from build123d import *

# Parameters (mm, degrees)
SKETCH2_R           = 145
SKETCH2_R_2         = 105
BOSS_EXTRUDE1_START = -50
SKETCH3_W           = 360
SKETCH3_H           = 360
SKETCH3_R           = 145
BOSS_EXTRUDE1_DEPTH = 50
FILLET1_R           = 20
SKETCH4_W           = 360
SKETCH4_H           = 360
SKETCH4_R           = 145
BOSS_EXTRUDE2_DEPTH = 50
FILLET2_R           = 20
SKETCH5_R           = 30
CUT_EXTRUDE1_DEPTH  = 10
CUT_EXTRUDE2_REACH  = 734.735
SKETCH6_R           = 15
CUT_EXTRUDE3_DEPTH  = 10
CUT_EXTRUDE4_REACH  = 848.699
SKETCH8_R           = 15
CIRPATTERN1_COUNT   = 4
CHAMFER1_SIZE       = 10
CHAMFER2_SIZE       = 10


with BuildPart() as part:
    # Sweep-Thin1: sweep along a path in Sketch1
    with BuildLine(Plane.XY) as sweep_thin1_path:
        Line((0, 0), (-150, 0))
        ThreePointArc((-150, 0), (-333.847763109, 76.152236891), (-410, 260))
        Line((-410, 260), (-410, 410))
    # Sketch2 → Sweep-Thin1 (sweep)
    with BuildSketch(Plane(origin=(0, 0, 0), x_dir=(0, 0, -1), z_dir=(1, 0, 0))):
        Circle(SKETCH2_R)
        Circle(SKETCH2_R_2, mode=Mode.SUBTRACT)
    sweep(path=sweep_thin1_path.line)

    # Sketch3 → Boss-Extrude1 (add)
    with BuildSketch(Plane(origin=(0, 0, 0), x_dir=(0, 0, -1), z_dir=(1, 0, 0)).offset(BOSS_EXTRUDE1_START)):
        Rectangle(SKETCH3_W, SKETCH3_H)
        with Locations(Location((0, 0, 0), (0, 0, 270))):
            Circle(SKETCH3_R, mode=Mode.SUBTRACT)
    extrude(amount=BOSS_EXTRUDE1_DEPTH)

    # Fillet1
    fillet1_edges = [part.edges().sort_by_distance(p)[0] for p in [
        (-25, -180, -180),
        (-25, -180, 180),
        (-25, 180, 180),
        (-25, 180, -180),
    ]]
    fillet(fillet1_edges, radius=FILLET1_R)

    # Sketch4 → Boss-Extrude2 (add)
    with BuildSketch(Plane(origin=(0, 410, 0), x_dir=(1, 0, 0), z_dir=(0, 1, 0))):
        with Locations((-410, 0)):
            Rectangle(SKETCH4_W, SKETCH4_H)
        with Locations(Location((-410, 0, 0), (0, 0, 180))):
            Circle(SKETCH4_R, mode=Mode.SUBTRACT)
    extrude(amount=-BOSS_EXTRUDE2_DEPTH)

    # Fillet2
    fillet2_edges = [part.edges().sort_by_distance(p)[0] for p in [
        (-230, 385, -180),
        (-230, 385, 180),
        (-590, 385, 180),
        (-590, 385, -180),
    ]]
    fillet(fillet2_edges, radius=FILLET2_R)

    # Sketch5 → Cut-Extrude1 (cut)
    with BuildSketch(Plane(origin=(0, 0, 0), x_dir=(0, 0, -1), z_dir=(1, 0, 0))):
        with Locations((-130, 130)):
            Circle(SKETCH5_R)
        with Locations((130, 130)):
            Circle(SKETCH5_R)
        with Locations((-130, -130)):
            Circle(SKETCH5_R)
        with Locations((130, -130)):
            Circle(SKETCH5_R)
    extrude(amount=-CUT_EXTRUDE1_DEPTH, mode=Mode.SUBTRACT)

    # Sketch6 → Cut-Extrude2 (cut, up to next)
    with BuildSketch(Plane(origin=(-10, 0, 0), x_dir=(0, 0, -1), z_dir=(1, 0, 0)), mode=Mode.PRIVATE) as cut_extrude2_sk1:
        with Locations((-130, 130)):
            Circle(SKETCH6_R)
    cut_extrude2_tool1 = extrude(cut_extrude2_sk1.sketch, amount=-CUT_EXTRUDE2_REACH, mode=Mode.PRIVATE) & part.part
    # Sketch6 → Cut-Extrude2 (cut, up to next)
    with BuildSketch(Plane(origin=(-10, 0, 0), x_dir=(0, 0, -1), z_dir=(1, 0, 0)), mode=Mode.PRIVATE) as cut_extrude2_sk2:
        with Locations(Location((130, 130, 0), (0, 0, 180))):
            Circle(SKETCH6_R)
    cut_extrude2_tool2 = extrude(cut_extrude2_sk2.sketch, amount=-CUT_EXTRUDE2_REACH, mode=Mode.PRIVATE) & part.part
    # Sketch6 → Cut-Extrude2 (cut, up to next)
    with BuildSketch(Plane(origin=(-10, 0, 0), x_dir=(0, 0, -1), z_dir=(1, 0, 0)), mode=Mode.PRIVATE) as cut_extrude2_sk3:
        with Locations((130, -130)):
            Circle(SKETCH6_R)
    cut_extrude2_tool3 = extrude(cut_extrude2_sk3.sketch, amount=-CUT_EXTRUDE2_REACH, mode=Mode.PRIVATE) & part.part
    # Sketch6 → Cut-Extrude2 (cut, up to next)
    with BuildSketch(Plane(origin=(-10, 0, 0), x_dir=(0, 0, -1), z_dir=(1, 0, 0)), mode=Mode.PRIVATE) as cut_extrude2_sk4:
        with Locations(Location((-130, -130, 0), (0, 0, 180))):
            Circle(SKETCH6_R)
    cut_extrude2_tool4 = extrude(cut_extrude2_sk4.sketch, amount=-CUT_EXTRUDE2_REACH, mode=Mode.PRIVATE) & part.part
    add(cut_extrude2_tool1.solids().sort_by_distance((-10, 130, 130))[0], mode=Mode.SUBTRACT)
    add(cut_extrude2_tool2.solids().sort_by_distance((-10, 130, -130))[0], mode=Mode.SUBTRACT)
    add(cut_extrude2_tool3.solids().sort_by_distance((-10, -130, -130))[0], mode=Mode.SUBTRACT)
    add(cut_extrude2_tool4.solids().sort_by_distance((-10, -130, 130))[0], mode=Mode.SUBTRACT)

    # Sketch7 → Cut-Extrude3 (cut)
    with BuildSketch(Plane(origin=(0, 410, 0), x_dir=(1, 0, 0), z_dir=(0, 1, 0))):
        with BuildLine():
            Line((-540, 100), (-540, 130))
            Line((-540, 130), (-510, 130))
            ThreePointArc((-510, 130), (-561.213203436, 151.213203436), (-540, 100))
        make_face()
        with BuildLine():
            Line((-510, 130), (-540, 130))
            Line((-540, 130), (-540, 100))
            ThreePointArc((-540, 100), (-518.786796564, 108.786796564), (-510, 130))
        make_face()
        with BuildLine():
            ThreePointArc((-250, 130), (-280, 160), (-310, 130))
            Line((-310, 130), (-280, 130))
            Line((-280, 130), (-280, 100))
            ThreePointArc((-280, 100), (-258.786796564, 108.786796564), (-250, 130))
        make_face()
        with BuildLine():
            Line((-280, 130), (-310, 130))
            ThreePointArc((-310, 130), (-301.213203436, 108.786796564), (-280, 100))
            Line((-280, 100), (-280, 130))
        make_face()
        with BuildLine():
            ThreePointArc((-250, -130), (-258.786796564, -108.786796564), (-280, -100))
            Line((-280, -100), (-280, -130))
            Line((-280, -130), (-310, -130))
            ThreePointArc((-310, -130), (-280, -160), (-250, -130))
        make_face()
        with BuildLine():
            Line((-280, -130), (-280, -100))
            ThreePointArc((-280, -100), (-301.213203436, -108.786796564), (-310, -130))
            Line((-310, -130), (-280, -130))
        make_face()
        with BuildLine():
            ThreePointArc((-510, -130), (-518.786796564, -108.786796564), (-540, -100))
            Line((-540, -100), (-540, -130))
            Line((-540, -130), (-510, -130))
        make_face()
        with BuildLine():
            Line((-540, -130), (-540, -100))
            ThreePointArc((-540, -100), (-561.213203436, -151.213203436), (-510, -130))
            Line((-510, -130), (-540, -130))
        make_face()
    extrude(amount=-CUT_EXTRUDE3_DEPTH, mode=Mode.SUBTRACT)

    # Sketch8 → Cut-Extrude4 (cut, up to next)
    with BuildSketch(Plane(origin=(0, 400, 0), x_dir=(1, 0, 0), z_dir=(0, 1, 0)), mode=Mode.PRIVATE) as cut_extrude4_sk1:
        with Locations(Location((-540, 130, 0), (0, 0, 180))):
            Circle(SKETCH8_R)
    cut_extrude4_tool1 = extrude(cut_extrude4_sk1.sketch, amount=-CUT_EXTRUDE4_REACH, mode=Mode.PRIVATE) & part.part
    cut_extrude4 = cut_extrude4_tool1.solids().sort_by_distance((-540, 400, -130))[0]
    add(cut_extrude4, mode=Mode.SUBTRACT)

    # CirPattern1: Cut-Extrude4 ×4 about axis
    cirpattern1_axis = Axis((-410, 0, 0), (0, 1, 0))
    for i in range(1, CIRPATTERN1_COUNT):
        add(cut_extrude4.rotate(cirpattern1_axis, i * 360 / CIRPATTERN1_COUNT), mode=Mode.SUBTRACT)

    # Chamfer1
    chamfer1_edges = [part.edges().sort_by_distance(p)[0] for p in [
        (0, 0, 105),
    ]]
    chamfer(chamfer1_edges, length=CHAMFER1_SIZE)

    # Chamfer2
    chamfer2_edges = [part.edges().sort_by_distance(p)[0] for p in [
        (-410, 410, 105),
    ]]
    chamfer(chamfer2_edges, length=CHAMFER2_SIZE)


solid = part.part
Can you work these out from the model? Positions are in its coordinate system, mm. A direction names the side the tool comes from. Give positions to 0.01 mm unless a question says otherwise; leave off trailing zeros. Write each loop counter-clockwise with the first axis right and the second up, starting at its lowest first coordinate (ties: lowest second). Pieces come first, ordered by that corner, then holes. Notation, with made-up numbers: (69, 76.5) -> (89, 76.5) arc R17 cw to (89, 98.5) -> close; hole circle Ø6 at (87, -19). An arc over 180 degrees is marked (long way). Answer as a JSON object with one key per item and string values. Group by question number.
Item 1: Suppose I cut it at A-A (z = 0). Please give me the cut outline in (x, y), plus the area to 3 significant figures.
Item 2: Suppose I cut it at C-C (x = -135). Please give me the cut outline in (y, z).
Item 3: For faces 4 (the face through (-534, 400, 116)), 5 (the face through (-453.554, 310.7, -138.304)), 6 (the face through (-10, -116, 124)), which set-ups out of +Z, -Z, +X, -X, +Y, -Y let a thin tool reach every point of the face, with its end or its side?
Item 4: Suppose I cut it at B-B (y = 130). State how many separate pieces and enclosed holes the cut face has, plus the area to 3 significant figures.
Item 5: I'm going to push flat-ended pins straight in: P1, Ø12, axis at x = -206, z = 90, coming from the -Y side; P2, Ø4, axis at x = -277.5, y = 332.5, coming from the -Z side; P3, Ø8, axis at x = -343.5, z = 89.5, coming from the -Y side. Where does each tip first touch, or does it pass through?
Item 6: Please list where these lines run through material, in increasing order: line 1 (Y direction, x = -3, z = -130); line 2 (X direction, y = 373, z = 130); line 3 (Z direction, x = -280, y = 381). Write a range as [from, to].
Item 7: We'd pull the mould along Z, two halves only. Please class faces 1 (the face through (-412, 385, -180)), 2 (the face through (-493, 410, -83)), 3 (the face through (-294.872, 380.28, -128.047)): +Z half, -Z half, draft (parallel to the pull), parting line (faces both ways), or undercut.
Item 8: Suppose I cut it at D-D (y = 273). Please give me the cut outline in (x, z).
Findings:
{
 "1": {"outline": "(-590, 360) -> (-555, 360) -> (-555, 260) arc R405 ccw to (-150, -145) -> (-50, -145) -> (-50, -180) -> (0, -180) -> (0, -115) -> (-10, -105) -> (-150, -105) arc R365 cw to (-515, 260) -> (-515, 400) -> (-525, 410) -> (-590, 410) -> close; (-305, 260) arc R155 ccw to (-150, 105) -> (-10, 105) -> (0, 115) -> (0, 180) -> (-50, 180) -> (-50, 145) -> (-150, 145) arc R115 cw to (-265, 260) -> (-265, 360) -> (-230, 360) -> (-230, 410) -> (-295, 410) -> (-305, 400) -> close", "area": "63,500 mm²"},
 "2": {"outline": "circle Ø290 at (0, 0); hole circle Ø210 at (0, 0)"},
 "3": {"face 4": "+Y", "face 5": "none", "face 6": "+X"},
 "4": {"separate pieces": "3", "enclosed holes": "1", "area": "71,600 mm²"},
 "5": {"P1": "stops at y = -114.11", "P2": "stops at z = -63.2", "P3": "stops at y = -64.43"},
 "6": {"line 1": "y = [-180, -160], [-100, 100], [160, 180]", "line 2": "x = [-590, -555], [-525, -295], [-265, -230]", "line 3": "z = [-180, -145], [-115, 115], [145, 180]"},
 "7": {"face 1": "-Z half", "face 2": "draft", "face 3": "undercut"},
 "8": {"outline": "circle Ø290 at (-410, 0); hole circle Ø210 at (-410, 0)"}
}
